from build123d import *

# Parameters (mm, degrees)
F0_W     = 65.9830570221
F0_H     = 45.4094596207
F1_DEPTH = 25.4


with BuildPart() as f1:
    # F0 (on Front) → F1 (new body)
    with BuildSketch(Plane.XZ):
        with Locations((-32.991528511, 22.7047298104)):
            Rectangle(F0_W, F0_H)
        Polygon((0, 45.4094596207), (0, 0), (26.1765359093, 26.0169209072), (32.039520707, 31.8441553545), align=None)
        Polygon((32.039520707, 31.8441553545), (26.1765359093, 26.0169209072), (53.0907474458, 22.9312162846), align=None)
    extrude(amount=F1_DEPTH)


solid = f1.part
Verification items for the finished model (mm, model axes). Coordinates: 2 decimals unless noted, no trailing zeros. Order: outer loops, then holes, each group sorted by start corner. A loop starts at its lowest first (then second) coordinate and runs counter-clockwise, first axis right, second up. Notation, with made-up numbers: (-23, 67.25) -> (-15, 67.25) arc R13 cw to (-15, 79.25) -> close; hole circle Ø10 at (29, 55). An arc over 180 degrees is marked (long way). Put each result on its own line as item: value. Start each with the question number.
1. Cross-section at A-A, the plane y = -10.25. Record the boundary of the cut face in (x, z), then the cut area to 3 significant figures.
2. Mould release check, pull along X, two halves, no side actions. Record for faces 1 (the flat face through (-65.983, -13, 22)), 2 (the flat face through (39.4, -12.5, 24.5)), 3 (the flat face through (-33, -13, 45.409)): released by +X, released by -X, zero draft, split by the parting line, or undercut.
3. Cross-section at B-B, the plane z = 34.5. Record the boundary of the cut face in (x, y).
4. Cross-section at C-C, the plane x = 46.5. Record the boundary of the cut face in (y, z).
5. Go/stop test with flat-tipped pins: pin 1 Ø2 at (x, z) = (29, 24) entering from +Y; pin 2 Ø5 at (x, y) = (29, -3.5) entering from +Z. Record where each tip stops, or that it passes through.
6. Material ranges on L1, parallel to X at y = -12, z = 34; L2, parallel to X at y = -4.75, z = 16; L3, parallel to Z at x = 4, y = -11, recorded low to high. Write a range as [from, to].
Computed:
1. outline: (-65.98, 0) -> (0, 0) -> (26.18, 26.02) -> (53.09, 22.93) -> (0, 45.41) -> (-65.98, 45.41) -> close
1. area: 3,810 mm2
2. face 1: released by -X
2. face 2: undercut
2. face 3: zero draft
3. outline: (-65.98, -25.4) -> (25.77, -25.4) -> (25.77, 0) -> (-65.98, 0) -> close
4. outline: (-25.4, 23.69) -> (0, 23.69) -> (0, 25.72) -> (-25.4, 25.72) -> close
5. pin 1: through
5. pin 2: z = 34.19
6. L1: [-65.98, 26.95]
6. L2: [-65.98, 16.1]
6. L3: [3.98, 43.72]
